The listing builds one solid part. Answer for the finished solid, in the listing's coordinates (mm). Face numbers are marked on the shaded views. Give positions to 0.01 mm unless a question says otherwise; leave off trailing zeros. Order: outer loops, then holes, each group sorted by start corner. A loop starts at its lowest first (then second) coordinate and runs counter-clockwise, first axis right, second up. Notation, with made-up numbers: (25, 81.5) -> (33, 81.5) arc R21 ccw to (33, 96.5) -> close; hole circle Ø1 at (-15, 32). An arc over 180 degrees is marked (long way). Answer as a JSON object with one key per item and string values. Group by question number.
```python
from build123d import *

# Parameters (mm, degrees)
EXTRUDE_1_DEPTH = 0.5


with BuildPart() as part:
    # Эскиз1 → Бобышка-Вытянуть1 (new body)
    with BuildSketch(Plane(origin=(0, 0, 0), x_dir=(1, 0, 0), z_dir=(0, 1, 0))):
        with BuildLine():
            Line((-0.5, 3.39653489), (-0.5, 3.617269734))
            Line((-0.5, 3.617269734), (-0.65, 3.617269734))
            ThreePointArc((-0.65, 3.617269734), (-1.383018397, 3.200677396), (-1.400206292, 2.357724418))
            ThreePointArc((-1.400206292, 2.357724418), (-1.350536641, 2.016782346), (-1.533211621, 1.724654938))
            ThreePointArc((-1.533211621, 1.724654938), (0, -2.75), (1.533211621, 1.724654938))
            ThreePointArc((1.533211621, 1.724654938), (1.350536641, 2.016782346), (1.400206292, 2.357724418))
            ThreePointArc((1.400206292, 2.357724418), (1.383018397, 3.200677396), (0.65, 3.617269734))
            Line((0.65, 3.617269734), (0.5, 3.617269734))
            Line((0.5, 3.617269734), (0.5, 3.39653489))
            ThreePointArc((0.5, 3.39653489), (0.532330319, 3.303508839), (0.615384615, 3.250583613))
            ThreePointArc((0.615384615, 3.250583613), (0.998565629, 2.801925275), (0.6875, 2.300566953))
            ThreePointArc((0.6875, 2.300566953), (0.551253141, 2.190164608), (0.5, 2.022459509))
            Line((0.5, 2.022459509), (0.5, 1.887458609))
            ThreePointArc((0.5, 1.887458609), (0.549878079, 1.72181132), (0.682926829, 1.611245154))
            ThreePointArc((0.682926829, 1.611245154), (0, -1.75), (-0.682926829, 1.611245154))
            ThreePointArc((-0.682926829, 1.611245154), (-0.549878079, 1.72181132), (-0.5, 1.887458609))
            Line((-0.5, 1.887458609), (-0.5, 2.022459509))
            ThreePointArc((-0.5, 2.022459509), (-0.551253141, 2.190164608), (-0.6875, 2.300566953))
            ThreePointArc((-0.6875, 2.300566953), (-0.998565629, 2.801925275), (-0.615384615, 3.250583613))
            ThreePointArc((-0.615384615, 3.250583613), (-0.532330319, 3.303508839), (-0.5, 3.39653489))
        make_face()
    extrude(amount=EXTRUDE_1_DEPTH)


solid = part.part
```
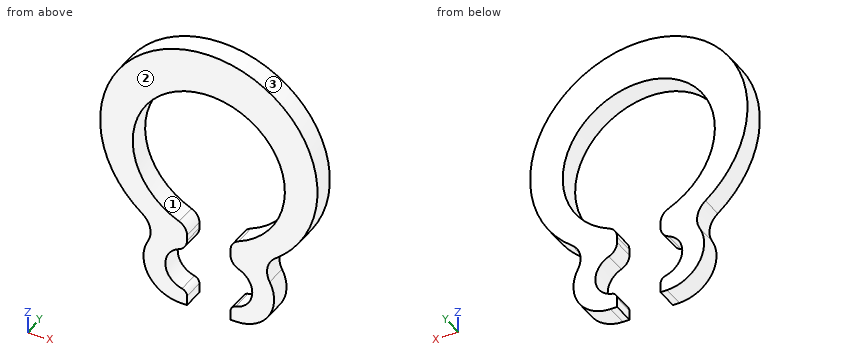
(1) A cutting plane is placed at D-D (z = 1.5). Determine the outline of the cut face in (x, y).
(2) For a pull along X with two mould halves and no side action, classify the marked faces 1, 2 and 3 as +X half, -X half, draft (parallel to the pull), parting line (faces both ways), or undercut.
(3) Find the intervals of material crossed by line 1 along Z through (x, y) = (0.9, 0.3); line 2 along X through (y, z) = (0.25, -3); line 3 along X through (y, z) = (0.15, 0.75), in increasing order. Write a range as [from, to].
(4) A cutting plane is placed at B-B (x = 0). Determine the outline of the cut face in (y, z), and give its area (3 significant figures).
(5) A cutting plane is placed at C-C (y = 0.3). Determine the outline of the cut face in (x, z).
(6) A cutting plane is placed at A-A (z = 0.25). Determine the outline of the cut face in (x, y).
(7) A flat-ended cylindrical pin translates along its axis: pin 1 Ø2 at (x, z) = (0.5, 2) entering from -Y. Find the tip coordinate at first contact, or state that the pin passes through.
Check sheet entries:
{
 "1": {"outline": "(-2.17, 0) -> (-0.9, 0) -> (-0.9, 0.5) -> (-2.17, 0.5) -> close; (0.9, 0) -> (2.17, 0) -> (2.17, 0.5) -> (0.9, 0.5) -> close"},
 "2": {"face 1": "undercut", "face 2": "draft", "face 3": "parting line"},
 "3": {"line 1": "z = [-3.58, -3.06], [-2.46, -1.5], [1.5, 2.58]", "line 2": "x = [-1.47, -0.94], [0.94, 1.47]", "line 3": "x = [-2.45, -1.58], [1.58, 2.45]"},
 "4": {"outline": "(0, 1.75) -> (0.5, 1.75) -> (0.5, 2.75) -> (0, 2.75) -> close", "area": "0.500 mm2"},
 "5": {"outline": "(-1.53, -1.72) arc R0.5 cw to (-1.4, -2.36) arc R0.85 ccw to (-0.65, -3.62) -> (-0.5, -3.62) -> (-0.5, -3.4) arc R0.15 ccw to (-0.62, -3.25) arc R0.5 cw to (-0.69, -2.3) arc R0.3 ccw to (-0.5, -2.02) -> (-0.5, -1.89) arc R0.3 ccw to (-0.68, -1.61) arc R1.75 cw (long way) to (0.68, -1.61) arc R0.3 ccw to (0.5, -1.89) -> (0.5, -2.02) arc R0.3 ccw to (0.69, -2.3) arc R0.5 cw to (0.62, -3.25) arc R0.15 ccw to (0.5, -3.4) -> (0.5, -3.62) -> (0.65, -3.62) arc R0.85 ccw to (1.4, -2.36) arc R0.5 cw to (1.53, -1.72) arc R2.5 ccw (long way) to start"},
 "6": {"outline": "(-2.5, 0) -> (-1.73, 0) -> (-1.73, 0.5) -> (-2.5, 0.5) -> close; (1.73, 0) -> (2.5, 0) -> (2.5, 0.5) -> (1.73, 0.5) -> close"},
 "7": {"pin 1": "stops at y = 0"}
}
